Geometry check sheet. Reference: the model listing, model coordinates, mm. Face numbers are marked on the shaded views. A direction names the side the tool comes from. Round coordinates to 2 decimals unless told otherwise and drop trailing zeros. Order: outer loops, then holes, each group sorted by start corner. A loop starts at its lowest first (then second) coordinate and runs counter-clockwise, first axis right, second up.
```python
from build123d import *

# Parameters (mm, degrees)
F0_W     = 89.221813
F0_H     = 41.016299
F1_DEPTH = 10
F2_W     = 8.577086
F2_H     = 2
F3_DEPTH = 41.017299
F4_W     = 3
F4_H     = 5.748613
F5_DEPTH = 41.017299


with BuildPart() as f1:
    # F0 (on Top) → F1 (new body)
    with BuildSketch(Plane.XY):
        with Locations((14.206558, -1.71161)):
            Rectangle(F0_W, F0_H)
    extrude(amount=F1_DEPTH)

    # F2 (on face) → F3 (cut, through all)
    with BuildSketch(Plane.XZ.offset(22.21976)):
        with Locations((54.528922, 1)):
            Rectangle(F2_W, F2_H)
    extrude(amount=-F3_DEPTH, mode=Mode.SUBTRACT)

    # F4 (on face) → F5 (cut, through all)
    with BuildSketch(Plane.XZ.offset(22.21976)):
        with Locations((-24.904348, 7.125694)):
            Rectangle(F4_W, F4_H)
        with Locations((-18.904348, 7.125694)):
            Rectangle(F4_W, F4_H)
        with Locations((-12.904348, 7.125694)):
            Rectangle(F4_W, F4_H)
        with Locations((-6.904348, 7.125694)):
            Rectangle(F4_W, F4_H)
        with Locations((-0.904348, 7.125694)):
            Rectangle(F4_W, F4_H)
        with Locations((5.095652, 7.125694)):
            Rectangle(F4_W, F4_H)
        with Locations((11.095652, 7.125694)):
            Rectangle(F4_W, F4_H)
        with Locations((17.095652, 7.125694)):
            Rectangle(F4_W, F4_H)
        with Locations((23.095652, 7.125694)):
            Rectangle(F4_W, F4_H)
        with Locations((29.095652, 7.125694)):
            Rectangle(F4_W, F4_H)
        with Locations((35.095652, 7.125694)):
            Rectangle(F4_W, F4_H)
        with Locations((41.095652, 7.125694)):
            Rectangle(F4_W, F4_H)
        with Locations((47.095652, 7.125694)):
            Rectangle(F4_W, F4_H)
        with Locations((53.095652, 7.125694)):
            Rectangle(F4_W, F4_H)
    extrude(amount=-F5_DEPTH, mode=Mode.SUBTRACT)


solid = f1.part
```
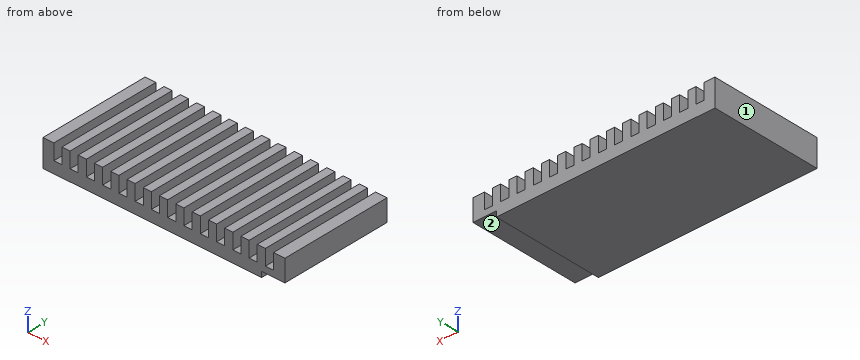
(1) Material ranges on line 1 (Z direction, x = -8, y = 2); line 2 (X direction, y = -16, z = 0.75), recorded low to high.
Returned:
line 1: z = 0 to 4.25
line 2: x = -30.4 to 50.24
(2) Sectioned sample at B-B, the plane x = 11.5. Record the cut outline in (y, z), and give its area (3 significant figures).
Returned:
outline: (-22.22, 0) - (18.8, 0) - (18.8, 4.25) - (-22.22, 4.25) - close
area: 174 mm2
(3) Set-up check for the marked faces 1 and 2: record each of +Z, -Z, +X, -X, +Y, -Y from which the full face is reachable in a straight line by a thin tool's end or side.
Returned:
face 1: +Z, -Z, -X, +Y, -Y
face 2: -Z, +X, +Y, -Y
(4) Depth check by flat-ended pin: P1, Ø3, axis at x = -6.5, y = -12, coming from the +Z side; P2, Ø0.6, axis at y = -6, z = 1.5, coming from the +X side; P3, Ø0.9, axis at x = -7, y = -5, coming from the +Z side. Enter the tip coordinate at first touch or a pass-through.
Returned:
P1: stops at z = 10
P2: stops at x = 50.24
P3: stops at z = 4.25
(5) Sectioned sample at A-A, the plane z = 6.5. Give the number of separate pieces and of enclosed holes in the cut face, and give its area (3 significant figures).
Returned:
separate pieces: 15
enclosed holes: 0
area: 1,940 mm2
